Verification items for the finished model (mm, model axes). Face numbers are marked on the shaded views. A direction names the side the tool comes from. Coordinates: 2 decimals unless noted, no trailing zeros. Order: outer loops, then holes, each group sorted by start corner. A loop starts at its lowest first (then second) coordinate and runs counter-clockwise, first axis right, second up. Notation, with made-up numbers: (-28, -2) -> (13, -2) arc R20 cw to (13, 36) -> close; hole circle Ø5 at (-7, 47). An arc over 180 degrees is marked (long way). Write each question's results on one line, items separated by ' | '. Start each with the question number.
(1) Cross-section at B-B on z = -9.5. Enter the section's corners in (x, y).
(2) Cross-section at D-D on x = 68. Enter the section's corners in (y, z), and give its area (3 significant figures).
(3) Go/stop test with flat-tipped pins: pin 1 (4 mm diameter, centred on y = 9.5, z = 1, fed in from +X); pin 2 (4.5 mm diameter, centred on y = 4, z = -35, fed in from -X); pin 3 (3.5 mm diameter, centred on x = -1, y = 3, fed in from -Z). Record where each tip stops, or that it passes through.
(4) Set-up check for the marked faces 1, 2, 3, 4 and 5: record each of +Z, -Z, +X, -X, +Y, -Y from which the full face is reachable in a straight line by a thin tool's end or side.
(5) Cross-section at A-A on x = 5.5. Enter the section's corners in (y, z), and give its area (3 significant figures).
(6) Thickness scan on probe 1 along X at (y, z) = (2.5, -22.5); probe 2 along X at (y, z) = (7.5, -35); probe 3 along Z at (x, y) = (10, 4). Record the ranges inside material, lowest first. Write a range as [from, to].
(7) Cross-section at C-C on x = 30.5. Enter the section's corners in (y, z).
```python
from build123d import *

# Parameters (mm, degrees)
SCHIZZO1_W                             = 28
SCHIZZO1_H                             = 48
ESTRUSIONE_ESTRUSIONE1_DEPTH           = 11
SCHIZZO3_R                             = 4.5
ESTRUSIONE_ESTRUSIONE2_DEPTH           = 12
SCHIZZO4_R                             = 4.5
ESTRUSIONE_ESTRUSIONE3_DEPTH           = 83.5
ESTRUSIONE_ESTRUSIONE3_TAPER           = 1
ESTRUSIONE_ESTRUSIONE3_OTHER_WAY_DEPTH = 4.5


with BuildPart() as part:
    # Schizzo1 → Estrusione-Estrusione1 (new body)
    with BuildSketch(Plane(origin=(0, 0, 0), x_dir=(1, 0, 0), z_dir=(0, 1, 0))):
        Rectangle(SCHIZZO1_W, SCHIZZO1_H)
    extrude(amount=ESTRUSIONE_ESTRUSIONE1_DEPTH)

    # Schizzo3 → Estrusione-Estrusione2 (add)
    with BuildSketch(Plane(origin=(0, 0, -24), x_dir=(-1, 0, 0), z_dir=(0, 0, -1))):
        with Locations(Location((8, 5.5, 0), (0, 0, 180))):
            Circle(SCHIZZO3_R)
    extrude(amount=ESTRUSIONE_ESTRUSIONE2_DEPTH)

    # Schizzo4 → Estrusione-Estrusione3 (add)
    with BuildSketch(Plane(origin=(-8, 0, 0), x_dir=(0, 0, -1), z_dir=(1, 0, 0))):
        with Locations((36, 5.5)):
            Circle(SCHIZZO4_R)
    extrude(amount=ESTRUSIONE_ESTRUSIONE3_DEPTH, taper=ESTRUSIONE_ESTRUSIONE3_TAPER)

    # Schizzo4 → Estrusione-Estrusione3 other way (add)
    with BuildSketch(Plane(origin=(-8, 0, 0), x_dir=(0, 0, -1), z_dir=(1, 0, 0))):
        with Locations((36, 5.5)):
            Circle(SCHIZZO4_R)
    extrude(amount=-ESTRUSIONE_ESTRUSIONE3_OTHER_WAY_DEPTH)


solid = part.part
```
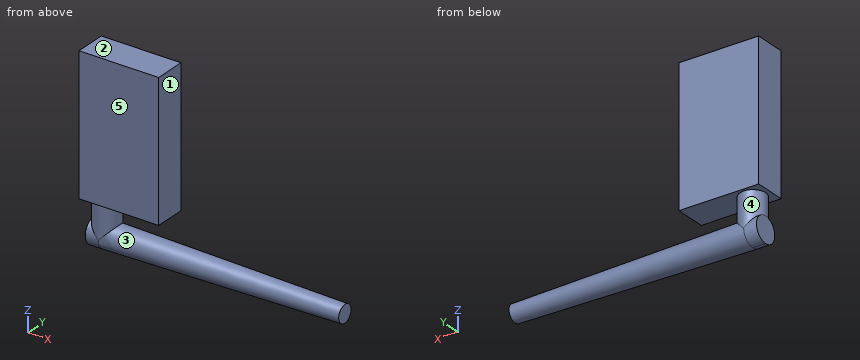
Results are:
1) outline: (-14, 0) -> (14, 0) -> (14, 11) -> (-14, 11) -> close
2) outline: circle Ø6.35 at (5.5, -36) | area: 31.6 mm2
3) pin 1: stops at x = 14 | pin 2: stops at x = -12.5 | pin 3: stops at z = -40.31
4) face 1: +Z, +X, +Y, -Y | face 2: +Z, +X, -X, +Y, -Y | face 3: +X | face 4: none | face 5: +Z, -Z, +X, -X, -Y
5) outline: (0, -24) -> (11, -24) -> (11, 24) -> (0, 24) -> close; circle Ø8.53 at (5.5, -36) | area: 585 mm2
6) probe 1: x = [-14, 14] | probe 2: x = [-12.5, 75.5] | probe 3: z = [-39.91, -32.09], [-24, 24]
7) outline: circle Ø7.66 at (5.5, -36)
